Here's how the part is built. I have some questions about the finished solid (model axes, mm). A direction names the side the tool comes from. Give positions to 0.01 mm unless a question says otherwise; leave off trailing zeros. Loops run counter-clockwise (first coordinate to the right, second up) from the corner with the lowest first, then second, coordinate; pieces in that order, holes last. Notation, with made-up numbers: (34, -40) - (60, -40) arc R26 cw to (60, -4) - close; hole circle Ø9 at (7.25, 48). An arc over 180 degrees is marked (long way). Use a Markdown table: item, result.
Autodesk Inventor part; units mm, degrees
ref_plane "YZ Plane" through (0, 0, 0) normal (1, 0, 0) x (0, 1, 0)
ref_plane "XZ Plane" through (0, 0, 0) normal (0, 1, 0) x (-1, 0, 0)
ref_plane "XY Plane" through (0, 0, 0) normal (0, 0, 1) x (1, 0, 0)
ref_plane "Work Plane1" through (-120.5056, -67.4861, 19.6827) normal (0, -1, 0) x (-0.7095338, 0, -0.7046714)
sketch "Sketch1" plane through (-120.5056, -67.4861, 19.6827) normal (0, -1, 0) x (-0.7095338, 0, -0.7046714)
  line L0 (-3.5869, -1.5817) -> (38.9131, -1.5817)
  line L1 (38.9131, -1.5817) -> (38.9131, 24.4183)
  line L2 (38.9131, 24.4183) -> (-3.5869, 24.4183)
  line L3 (-3.5869, 24.4183) -> (-3.5869, -1.5817)
  point P0 (-71.6329, 98.8824)
  dimension "d0" = 42.5
  dimension "d1" = 26
extrude "Extrusion1" add sketch "Sketch1" against normal blind 24
shell "Shell1" thickness 6 removed faces 1 at (-129.1269, -59.4861, 13.3497)
sketch "Sketch2" plane through (-119.0751, -67.4861, 23.3326) normal (-0.7046714, 0, 0.7095338) x (0.7095338, 0, 0.7046714)
  line L0 (0, 0) -> (-42.5, 0)
  line L1 (-42.5, 0) -> (-42.5, 24)
  line L2 (0, 0) -> (-42.5, 0)
  line L3 (-42.5, 0) -> (-42.5, 5)
  line L4 (-42.5, 5) -> (0, 5)
  line L5 (0, 5) -> (0, 0)
  line L6 (0, 24) -> (-42.5, 24)
  line L7 (-42.5, 24) -> (-42.5, 19)
  line L8 (-42.5, 19) -> (0, 19)
  line L9 (0, 19) -> (0, 24)
  point P0 (68.046, 67.4861)
  dimension "d5" = 5
  dimension "d7" = 5
extrude "Extrusion2" cut sketch "Sketch2" against normal through all
sketch "Sketch3" plane through (-119.0751, -62.4861, 23.3326) normal (0, -1, 0) x (-0.7095338, 0, -0.7046714)
  line L0 (42.5, 26) -> (42.5, 0)
  line L1 (0, 26) -> (42.5, 26)
  line L2 (42.5, 26) -> (42.5, 21)
  line L3 (42.5, 21) -> (0, 21)
  line L4 (0, 21) -> (0, 26)
  point P0 (-68.046, 100.4641)
  dimension "d10" = 5
extrude "Extrusion3" cut sketch "Sketch3" against normal through all
properties part number "ServoHolder"
(1) On a 3-axis mill with a long thin cutter (end or side, diameter ignored), from which of +Z, -Z, +X, -X, +Y, -Y can I reach the whole of each face in a straight line? I mean faces 4 (the face through (-116.187, -55.57, 11.91)), 5 (the face through (-120.21, -55.57, -5.98)), 6 (the face through (-127, -48.486, 1)). Say none if no direction works.
A:
| item | result |
|---|---|
| face 4 | -X |
| face 5 | none |
| face 6 | +Z, -Z, +X, -X, +Y |
(2) Suppose I cut it at D-D on y = -55.5. Write out the boundary of the cut face in (x, z), plus the area to 4 significant figures.
A:
| item | result |
|---|---|
| outline | (-149.23, -6.62) - (-134.43, -21.52) - (-104.28, 8.43) - (-119.08, 23.33) - (-123.33, 19.1) - (-109.24, 4.91) - (-130.88, -16.58) - (-144.97, -2.39) - close |
| area | 282.5 mm2 |
(3) If I drill on line 1 (Y direction, x = -119, z = 14); line 2 (Z direction, x = -115, y = -52.75); line 3 (X direction, y = -50.75, z = -11.5), over which ranges is the centre line in solid material (lowest first)?
A:
| item | result |
|---|---|
| line 1 | -62.49 to -61.49, -49.49 to -48.49 |
| line 2 | -2.22 to -0.81, 10.71 to 19.23 |
| line 3 | -144.38 to -135.92, -125.77 to -124.35 |
(4) Will these pins go through, and if not, where does the flat tip stop? pin 1 (5 mm diameter, centred on y = -50.5, z = 3.5, fed in from +X); pin 2 (3 mm diameter, centred on y = -58.5, z = -16, fed in from -X); pin 3 (1.5 mm diameter, centred on x = -137.5, y = -55.5, fed in from -Z).
A:
| item | result |
|---|---|
| pin 1 | x = -106.73 |
| pin 2 | x = -141.4 |
| pin 3 | z = -19.18 |
(5) We'd pull the mould along Y, two halves only. Please class faces 1 (the face through (-119.566, -55.584, -6.752)), 2 (the face through (-127, -62.486, 1)), 3 (the face through (-138.03, -55.57, -9.38)): pulls with the +Y half, pulls with the -Y half, needs draft (parallel to the pull), parting line crosses it, or undercut.
A:
| item | result |
|---|---|
| face 1 | needs draft |
| face 2 | pulls with the -Y half |
| face 3 | undercut |
(6) Suppose I cut it at A-A on x = -117. Write out the boundary of the cut face in (y, z).
A:
| item | result |
|---|---|
| outline | (-62.49, -4.2) - (-48.49, -4.2) - (-48.49, 21.24) - (-62.49, 21.24) - close; hole (-61.49, -2.79) - (-49.49, -2.79) - (-49.49, 12.73) - (-61.49, 12.73) - close |
(7) Suppose I cut it at C-C on z = 7.5. Write out the boundary of the cut face in (x, y).
A:
| item | result |
|---|---|
| outline | (-135.02, -62.49) - (-105.22, -62.49) - (-105.22, -48.49) - (-135.02, -48.49) - (-135.02, -49.49) - (-111.81, -49.49) - (-111.81, -61.49) - (-135.02, -61.49) - close |
(8) Suppose I cut it at B-B on z = -15.5. Write out the boundary of the cut face in (x, y).
A:
| item | result |
|---|---|
| outline | (-140.41, -62.49) - (-128.37, -62.49) - (-128.37, -48.49) - (-140.41, -48.49) - close; hole (-131.95, -61.49) - (-129.79, -61.49) - (-129.79, -49.49) - (-131.95, -49.49) - close |
